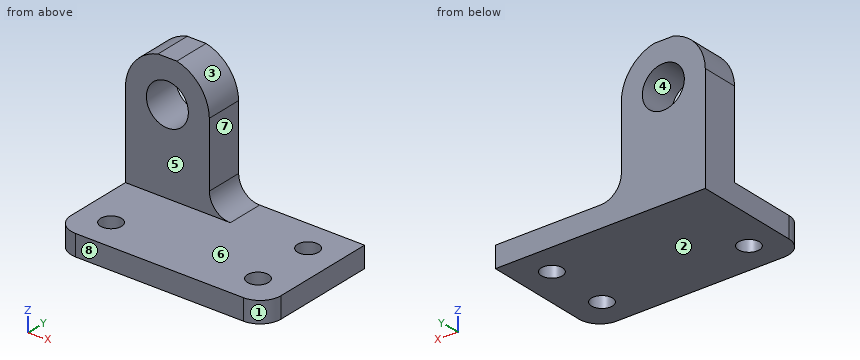
```python
from build123d import *

# Parameters (mm, degrees)
F1_DEPTH = 63.5
F3_DEPTH = 12.7
F4_R     = 6.35
F5_DEPTH = 12.7
F6_R     = 3.175
F7_DEPTH = 6.35


with BuildPart() as f1:
    # F0 (on Right) → F1 (new body)
    with BuildSketch(Plane.YZ):
        Polygon((0, 6.35), (0, 0), (38.1, 0), (38.1, 44.45), (26.9596510282, 44.45), (26.9596510282, 6.35), align=None)
    extrude(amount=F1_DEPTH)

    # F2 (on face) → F3 (cut)
    with BuildSketch(Plane.XZ.offset(-26.9596510282)):
        with BuildLine():
            Line((63.5, 44.45), (25.4, 44.45))
            Line((25.4, 44.45), (25.4, 12.7))
            ThreePointArc((25.4, 12.7), (27.2598719395, 8.2098719395), (31.75, 6.35))
            Line((31.75, 6.35), (63.5, 6.35))
            Line((63.5, 6.35), (63.5, 44.45))
        make_face()
    extrude(amount=-F3_DEPTH, mode=Mode.SUBTRACT)

    # F4 (on face) → F5 (cut)
    with BuildSketch(Plane.XZ.offset(-26.9596510282)):
        with BuildLine():
            ThreePointArc((15.5470193775, 44.45), (22.5386496815, 40.1060799579), (25.4, 32.3882298689))
            Line((25.4, 32.3882298689), (25.4, 44.45))
            Line((25.4, 44.45), (15.5470193775, 44.45))
        make_face()
        with Locations((12.7, 31.75)):
            Circle(F4_R)
        with BuildLine():
            ThreePointArc((0, 32.3882298689), (2.8613503185, 40.1060799579), (9.8529806225, 44.45))
            Line((9.8529806225, 44.45), (0, 44.45))
            Line((0, 44.45), (0, 32.3882298689))
        make_face()
    extrude(amount=-F5_DEPTH, mode=Mode.SUBTRACT)

    # F6 (on face) → F7 (cut)
    with BuildSketch(Plane.XY.offset(6.35)):
        with Locations((53.975, 9.525)):
            Circle(F6_R)
        with BuildLine():
            ThreePointArc((63.5, 6.35), (61.6401280605, 1.8598719395), (57.15, 0))
            Line((57.15, 0), (63.5, 0))
            Line((63.5, 0), (63.5, 6.35))
        make_face()
        with BuildLine():
            ThreePointArc((6.35, 0), (1.8598719395, 1.8598719395), (0, 6.35))
            Line((0, 6.35), (0, 0))
            Line((0, 0), (6.35, 0))
        make_face()
        with Locations((9.525, 9.525)):
            Circle(F6_R)
        with Locations((53.975, 28.575005229)):
            Circle(F6_R)
    extrude(amount=-F7_DEPTH, mode=Mode.SUBTRACT)


solid = f1.part
```
Geometry check sheet. Reference: the model listing, model coordinates, mm. Face numbers are marked on the shaded views. A direction names the side the tool comes from. Round coordinates to 2 decimals unless told otherwise and drop trailing zeros. Order: outer loops, then holes, each group sorted by start corner. A loop starts at its lowest first (then second) coordinate and runs counter-clockwise, first axis right, second up. Notation, with made-up numbers: (26, 88.5) - (48, 88.5) arc R33 ccw to (48, 116.5) - close; hole circle Ø9 at (89.25, 49). An arc over 180 degrees is marked (long way). Use a Markdown table: item, result. Add a question column.
1) Thickness scan on line 1 along Z through (x, y) = (12.7, 34); line 2 along X through (y, z) = (27, 15.5); line 3 along Y through (x, z) = (12.5, 41). Record the ranges inside material, lowest first.
2) Section check B-B (z = 27). Record the cut outline in (x, y), then the cut area to 3 significant figures.
3) Section check D-D (x = 36.5). Record the cut outline in (y, z).
4) Mould release check, pull along Z, two halves, no side actions. Record for the marked faces 1, 2, 3 and 4: released by +Z, released by -Z, zero draft, split by the parting line, or undercut.
5) Gauge pin test, flat ends, axial feed: P1, Ø9.5, axis at x = 9, z = 22.5, coming from the -Y side; P2, Ø3.5, axis at y = 32, z = 23.5, coming from the +X side; P3, Ø11.5, axis at x = 16, y = 10, coming from the +Z side; P4, Ø11.5, axis at x = 12.7, z = 31.75, coming from the -Y side. Record the tip position at first contact, or that the pin passes through.
6) Set-up check for the marked faces 5, 6, 7 and 8: record each of +Z, -Z, +X, -X, +Y, -Y from which the full face is reachable in a straight line by a thin tool's end or side.
7) Section check C-C (z = 5.5). Record the cut outline in (x, y) (3 decimals), then the cut area to 3 significant figures.
8) Section check A-A (x = 51.5). Record the cut outline in (y, z).
Established:
| question | item | result |
|---|---|---|
| 1 | line 1 | 0 to 25.4, 38.1 to 44.45 |
| 1 | line 2 | 0 to 25.4 |
| 1 | line 3 | 26.96 to 38.1 |
| 2 | outline | (0, 26.96) - (8.49, 26.96) - (8.49, 38.1) - (0, 38.1) - close; (16.91, 26.96) - (25.4, 26.96) - (25.4, 38.1) - (16.91, 38.1) - close |
| 2 | area | 189 mm2 |
| 3 | outline | (0, 0) - (38.1, 0) - (38.1, 6.35) - (0, 6.35) - close |
| 4 | face 1 | zero draft |
| 4 | face 2 | released by -Z |
| 4 | face 3 | released by +Z |
| 4 | face 4 | undercut |
| 5 | P1 | y = 26.96 |
| 5 | P2 | x = 25.4 |
| 5 | P3 | z = 6.35 |
| 5 | P4 | through |
| 6 | face 5 | +Z, +X, -X, -Y |
| 6 | face 6 | +Z, +X, -Y |
| 6 | face 7 | +Z, +X, +Y, -Y |
| 6 | face 8 | +Z, -Z, +X, -X, -Y |
| 7 | outline | (0, 6.35) arc R6.35 ccw to (6.35, 0) - (57.15, 0) arc R6.35 ccw to (63.5, 6.35) - (63.5, 38.1) - (0, 38.1) - close; hole circle Ø6.35 at (9.525, 9.525); hole circle Ø6.35 at (53.975, 9.525); hole circle Ø6.35 at (53.975, 28.575) |
| 7 | area | 2,310 mm2 |
| 8 | outline | (0, 0) - (7.54, 0) - (7.54, 6.35) - (0, 6.35) - close; (11.51, 0) - (26.59, 0) - (26.59, 6.35) - (11.51, 6.35) - close; (30.56, 0) - (38.1, 0) - (38.1, 6.35) - (30.56, 6.35) - close |
